The listing builds one solid part. Answer for the finished solid, in the listing's coordinates (mm). Coordinates: 2 decimals unless noted, no trailing zeros. Order: outer loops, then holes, each group sorted by start corner. A loop starts at its lowest first (then second) coordinate and runs counter-clockwise, first axis right, second up. Notation, with made-up numbers: (81, 6) -> (101, 6) arc R10 cw to (101, 20) -> close; hole circle Ø4 at (23.5, -5.5). An arc over 180 degrees is marked (long way). Write each question's results on one line, items separated by ' | '. Start each with the question number.
(1) Straight lines are drawn through the part: L1, parallel to Y at x = 157, z = 1.95; L2, parallel to X at y = 119, z = 1.7; L3, parallel to X at y = 76.5, z = 0.85. For each, find the intervals that lie inside material, in ascending order.
(2) The part is cut by section A-A, the plane x = 147.5. Give the vertices of the cut face in (y, z).
(3) The part is cut by section B-B, the plane y = 115. Give the vertices of the cut face in (x, z).
(4) The part is cut by section C-C, the plane z = 0.9. Count the separate pieces of the cut face and the enclosed holes in it, then the cut area to 3 significant figures.
(5) Given pin 1 (0.6 mm diameter, centred on x = 102, z = 1, fed in from -Y); pin 2 (1.6 mm diameter, centred on x = 96.68, y = 107.26, fed in from -Z); pin 3 (1 mm diameter, centred on x = 100.5, z = 1, fed in from +Y), each flat-ended and moving along its own axis, determine where each tip first touches the part or whether it passes through.
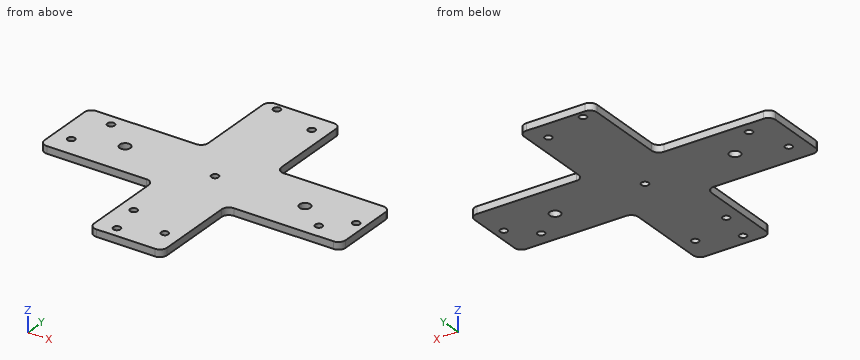
```python
from build123d import *

# Parameters (mm, degrees)
SKETCH_3_R      = 1.5
SKETCH_3_R_2    = 1
EXTRUDE_1_DEPTH = 2


with BuildPart() as part:
    # 草图3 → 凸台-拉伸1 (new body)
    with BuildSketch(Plane.XY):
        with BuildLine():
            Line((118.06282276, 110.61097636), (90.364678066, 110.61097636))
            ThreePointArc((90.364678066, 110.61097636), (88.950464504, 110.025189922), (88.364678066, 108.61097636))
            Line((88.364678066, 108.61097636), (88.364678066, 92.490482591))
            ThreePointArc((88.364678066, 92.490482591), (88.950464504, 91.076269028), (90.364678066, 90.490482591))
            Line((90.364678066, 90.490482591), (118.06282276, 90.490482591))
            ThreePointArc((118.06282276, 90.490482591), (119.477036322, 89.904696153), (120.06282276, 88.490482591))
            Line((120.06282276, 88.490482591), (120.06282276, 66.422251235))
            ThreePointArc((120.06282276, 66.422251235), (120.648609197, 65.008037673), (122.06282276, 64.422251235))
            Line((122.06282276, 64.422251235), (138.340493265, 64.422251235))
            ThreePointArc((138.340493265, 64.422251235), (139.754706828, 65.008037673), (140.340493265, 66.422251235))
            Line((140.340493265, 66.422251235), (140.340493265, 88.490482591))
            ThreePointArc((140.340493265, 88.490482591), (140.926279703, 89.904696153), (142.340493265, 90.490482591))
            Line((142.340493265, 90.490482591), (170.038637959, 90.490482591))
            ThreePointArc((170.038637959, 90.490482591), (171.452851521, 91.076269028), (172.038637959, 92.490482591))
            Line((172.038637959, 92.490482591), (172.038637959, 108.61097636))
            ThreePointArc((172.038637959, 108.61097636), (171.452851521, 110.025189922), (170.038637959, 110.61097636))
            Line((170.038637959, 110.61097636), (142.340493265, 110.61097636))
            ThreePointArc((142.340493265, 110.61097636), (140.926279703, 111.196762797), (140.340493265, 112.61097636))
            Line((140.340493265, 112.61097636), (140.340493265, 134.679207715))
            ThreePointArc((140.340493265, 134.679207715), (139.754706828, 136.093421277), (138.340493265, 136.679207715))
            Line((138.340493265, 136.679207715), (122.06282276, 136.679207715))
            ThreePointArc((122.06282276, 136.679207715), (120.648609197, 136.093421277), (120.06282276, 134.679207715))
            Line((120.06282276, 134.679207715), (120.06282276, 112.61097636))
            ThreePointArc((120.06282276, 112.61097636), (119.477036322, 111.196762797), (118.06282276, 110.61097636))
        make_face()
        with Locations((105.201658013, 100.550729475)):
            Circle(SKETCH_3_R, mode=Mode.SUBTRACT)
        with Locations(Location((155.201658013, 100.550729475, 0), (0, 0, 180))):
            Circle(SKETCH_3_R, mode=Mode.SUBTRACT)
        with Locations((136.017880342, 131.156826246)):
            Circle(SKETCH_3_R_2, mode=Mode.SUBTRACT)
        with Locations((123.959858439, 76.753868602)):
            Circle(SKETCH_3_R_2, mode=Mode.SUBTRACT)
        with Locations((93.105508276, 96.40135135)):
            Circle(SKETCH_3_R_2, mode=Mode.SUBTRACT)
        with Locations((169.425693967, 100.550729475)):
            Circle(SKETCH_3_R_2, mode=Mode.SUBTRACT)
        with Locations((130.201658013, 100.550729475)):
            Circle(SKETCH_3_R_2, mode=Mode.SUBTRACT)
        with Locations((125.650168223, 67.53399009)):
            Circle(SKETCH_3_R_2, mode=Mode.SUBTRACT)
        with Locations((123.959858439, 134.679207715)):
            Circle(SKETCH_3_R_2, mode=Mode.SUBTRACT)
        with Locations((96.683392317, 107.263125424)):
            Circle(SKETCH_3_R_2, mode=Mode.SUBTRACT)
        with Locations((163.089439849, 94.66887503)):
            Circle(SKETCH_3_R_2, mode=Mode.SUBTRACT)
        with Locations((136.017880342, 71.77023795)):
            Circle(SKETCH_3_R_2, mode=Mode.SUBTRACT)
    extrude(amount=EXTRUDE_1_DEPTH)


solid = part.part
```
Established:
1) L1: y = 90.49 to 110.61 | L2: x = 120.06 to 140.34 | L3: x = 120.06 to 122.99, 124.93 to 140.34
2) outline: (90.49, 0) -> (110.61, 0) -> (110.61, 2) -> (90.49, 2) -> close
3) outline: (120.06, 0) -> (140.34, 0) -> (140.34, 2) -> (120.06, 2) -> close
4) separate pieces: 1 | enclosed holes: 12 | area: 2,690 mm^2
5) pin 1: stops at y = 90.49 | pin 2: passes through | pin 3: stops at y = 110.61
